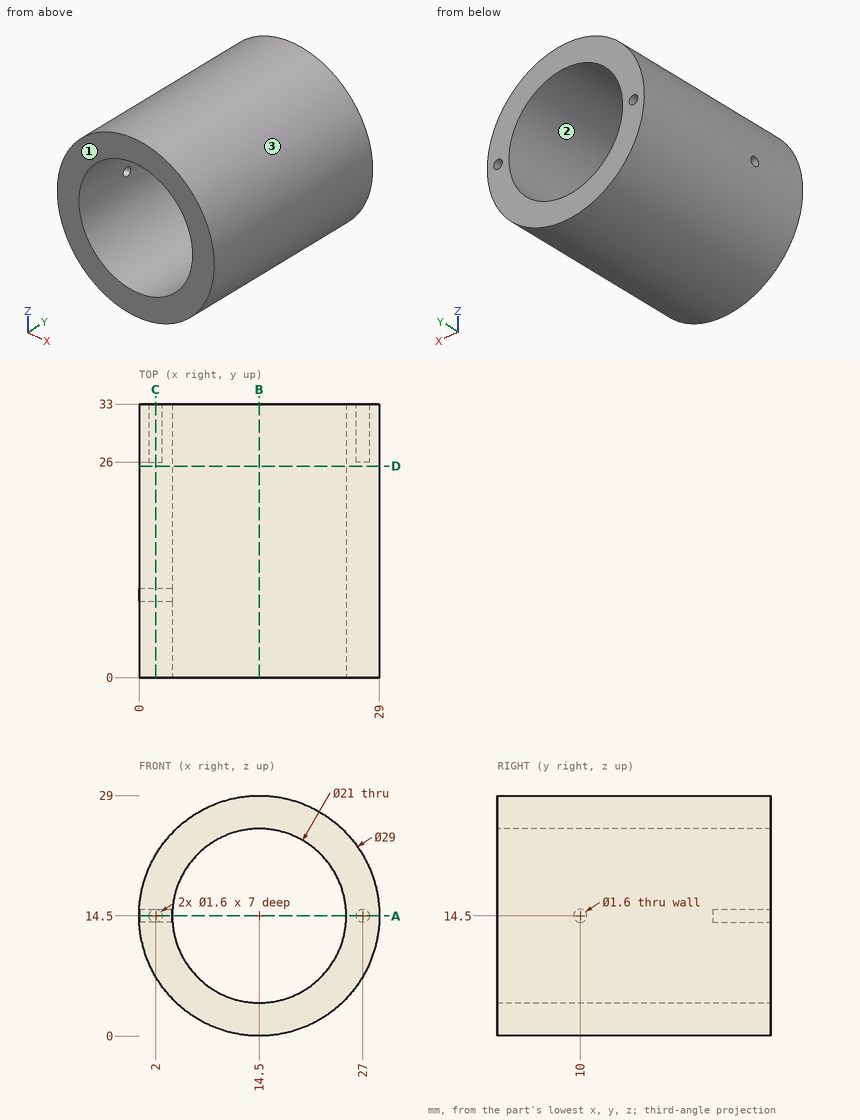
Geometry: see drawing. Coordinates: mm, zero at the bounding-box minimum. Round coordinates to 2 decimals unless told otherwise and drop trailing zeros. Loops run counter-clockwise (first coordinate to the right, second up) from the corner with the lowest first, then second, coordinate; pieces in that order, holes last. Notation, with made-up numbers: M 70.5,60 L 97.5,60 A29 ccw 97.5,92 Z; hole C 4.25,-22 d5. An arc over 180 degrees is marked long. Use a Markdown table: item, result. Add a question column.
1. Cut plane D-D, the plane y = 25.5. Output: boundary loops of the cut face in (x, z).
2. Pull-direction query (X, two-part tool) for the marked faces 1, 2 and 3; classes: +X half, -X half, draft (parallel to the pull), parting line (faces both ways), or undercut.
3. Cut plane B-B, the plane x = 14.5. Output: boundary loops of the cut face in (y, z), and give its area (3 significant figures).
4. Cut plane C-C, the plane x = 2. Output: boundary loops of the cut face in (y, z).
5. Cut plane A-A, the plane z = 14.5. Output: boundary loops of the cut face in (x, y).
6. Ray query, line 1 along X through (y, z) = (11, 14.5); line 2 along X through (y, z) = (15.5, 23.5); line 3 along Z through (x, y) = (27, 30.75). Return the intervals inside material, ascending. Write a range as [from, to].
7. Contact query for flat-ended pins moving along their axis: pin 1 (1.3 mm diameter, centred on x = 27, z = 14, fed in from +Y); pin 2 (1.4 mm diameter, centred on x = 2, z = 14.5, fed in from +Y); pin 3 (1 mm diameter, centred on x = 6, y = 22, fed in from +Z); pin 4 (2 mm diameter, centred on y = 9.5, z = 21.5, fed in from -X). Output: stop coordinate, or through.
Solution:
| question | item | result |
|---|---|---|
| 1 | outline | C 14.5,14.5 d29; hole C 14.5,14.5 d21 |
| 2 | face 1 | draft |
| 2 | face 2 | undercut |
| 2 | face 3 | parting line |
| 3 | outline | M 0,0 L 33,0 L 33,4 L 0,4 Z; M 0,25 L 33,25 L 33,29 L 0,29 Z |
| 3 | area | 264 mm2 |
| 4 | outline | M 0,7.15 L 33,7.15 L 33,13.7 L 26,13.7 L 26,15.3 L 33,15.3 L 33,21.85 L 0,21.85 Z; hole C 10,14.5 d1.6 |
| 5 | outline | M 0,0 L 4,0 L 4,9.2 L 0,9.2 Z; M 0,10.8 L 4,10.8 L 4,33 L 2.8,33 L 2.8,26 L 1.2,26 L 1.2,33 L 0,33 Z; M 25,0 L 29,0 L 29,33 L 27.8,33 L 27.8,26 L 26.2,26 L 26.2,33 L 25,33 Z |
| 6 | line 1 | x = [0, 4], [25, 29] |
| 6 | line 2 | x = [3.13, 9.09], [19.91, 25.87] |
| 6 | line 3 | z = [7.15, 13.7], [15.3, 21.85] |
| 7 | pin 1 | stops at y = 33 |
| 7 | pin 2 | stops at y = 26 |
| 7 | pin 3 | stops at z = 26.59 |
| 7 | pin 4 | stops at x = 1.3 |
